from build123d import *

# Parameters (mm, degrees)
SKETCH1_R           = 2
BOSS_EXTRUDE1_DEPTH = 6
SKETCH2_R           = 10
BOSS_EXTRUDE2_DEPTH = 51
SKETCH3_R           = 7.75
CUT_EXTRUDE1_DEPTH  = 62.558024733
FILLET1_R           = 1


with BuildPart() as part:
    # Sketch1 → Boss-Extrude1 (new body)
    with BuildSketch(Plane(origin=(0, 0, 0), x_dir=(1, 0, 0), z_dir=(0, 1, 0))):
        Polygon((-16.274775851, 13.401142209), (-14.274775851, 15.401142209), (13.725224149, 15.401142209), (15.725224149, 13.401142209), (15.725224149, -14.598857791), (13.725224149, -16.598857791), (-14.274775851, -16.598857791), (-16.274775851, -14.598857791), align=None)
        with Locations(Location((11.038932647, 10.714850708, 0), (0, 0, 270))):
            Circle(SKETCH1_R, mode=Mode.SUBTRACT)
        with Locations(Location((-11.58848435, 10.714850708, 0), (0, 0, 270))):
            Circle(SKETCH1_R, mode=Mode.SUBTRACT)
        with Locations(Location((-11.58848435, -11.91256629, 0), (0, 0, 270))):
            Circle(SKETCH1_R, mode=Mode.SUBTRACT)
        with Locations(Location((11.038932647, -11.91256629, 0), (0, 0, 270))):
            Circle(SKETCH1_R, mode=Mode.SUBTRACT)
    extrude(amount=BOSS_EXTRUDE1_DEPTH)

    # Sketch2 → Boss-Extrude2 (add)
    with BuildSketch(Plane(origin=(0, 6, 0), x_dir=(1, 0, 0), z_dir=(0, 1, 0))):
        with Locations(Location((-0.274775851, -0.598857791, 0), (0, 0, 90))):
            Circle(SKETCH2_R)
    extrude(amount=BOSS_EXTRUDE2_DEPTH)

    # Sketch3 → Cut-Extrude1 (cut, through all)
    with BuildSketch(Plane(origin=(0, 57, 0), x_dir=(1, 0, 0), z_dir=(0, 1, 0))):
        with Locations(Location((-0.274775851, -0.598857791, 0), (0, 0, 270))):
            Circle(SKETCH3_R)
    extrude(amount=-CUT_EXTRUDE1_DEPTH, mode=Mode.SUBTRACT)

    # Fillet1
    fillet1_edges = [part.edges().sort_by_distance(p)[0] for p in [
        (-0.274775851, 6, 10.598857791),
    ]]
    fillet(fillet1_edges, radius=FILLET1_R)


solid = part.part
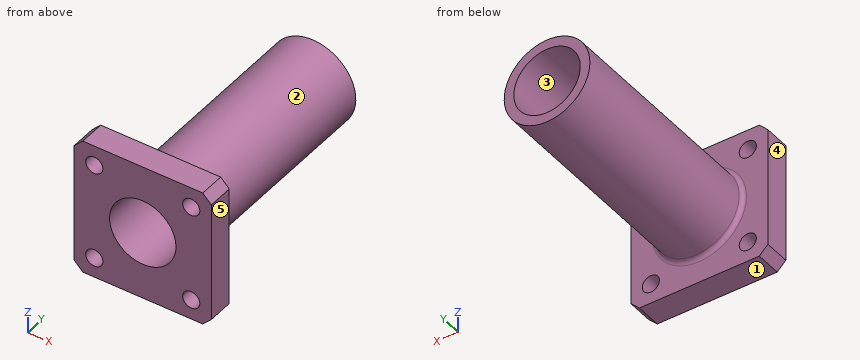
Could you check a few things on this model? Use its own coordinates, in mm. Face numbers are marked on the shaded views. A direction names the side the tool comes from. Coordinates: 2 decimals unless noted, no trailing zeros. Order: outer loops, then holes, each group sorted by start corner. A loop starts at its lowest first (then second) coordinate and runs counter-clockwise, first axis right, second up. Notation, with made-up numbers: (43.5, -34.5) - (57.5, -34.5) arc R21 cw to (57.5, -0.5) - close; hole circle Ø11 at (81, -15.5). An arc over 180 degrees is marked (long way). Answer in a Markdown table with one row per item. Add a question column.
(1) If we mould it in two halves opening along X, with no side actions, what happens to the marked faces 3, 4 and 5? For each: released by +X, released by -X, zero draft, split by the parting line, or undercut.
(2) If we section it at A-A, the plane x = -12.5: Please give me the cut outline in (y, z), then the cut area to 3 significant figures.
(3) Will these pins go through, and if not, where does the flat tip stop? pin 1 (2.5 mm diameter, centred on x = 11.04, z = 11.91, fed in from -Y); pin 2 (2 mm diameter, centred on y = 28.5, z = 7, fed in from -X); pin 3 (1.5 mm diameter, centred on y = 38.5, z = 3.5, fed in from -X); pin 4 (4 mm diameter, centred on y = 27, z = -10.5, fed in from -X).
(4) I need wall thicknesses on L1, parallel to Z at x = 0, y = 4; L2, parallel to X at y = 45, z = 1; L3, parallel to Y at x = 5, z = -11. Which ranges of each line are inside material? Lowest first, please.
(5) If we section it at B-B, the plane y = 21.5: Please give me the cut outline in (x, z), then the cut area to 3 significant figures.
(6) On a 3-axis mill with a long thin cutter (end or side, diameter ignored), from which of +Z, -Z, +X, -X, +Y, -Y can I reach the whole of each face in a straight line? I mean the marked faces 1 and 2. Say none if no direction works.
Results are:
| question | item | result |
|---|---|---|
| 1 | face 3 | undercut |
| 1 | face 4 | released by -X |
| 1 | face 5 | released by +X |
| 2 | outline | (0, -15.4) - (6, -15.4) - (6, -12.5) - (0, -12.5) - close; (0, -8.93) - (6, -8.93) - (6, 10.13) - (0, 10.13) - close; (0, 13.69) - (6, 13.69) - (6, 16.6) - (0, 16.6) - close |
| 2 | area | 149 mm2 |
| 3 | pin 1 | passes through |
| 3 | pin 2 | stops at x = -8.69 |
| 3 | pin 3 | stops at x = -10.04 |
| 3 | pin 4 | stops at x = -4.42 |
| 4 | L1 | z = -15.4 to -7.15, 8.34 to 16.6 |
| 4 | L2 | x = -10.27 to -8.01, 7.46 to 9.72 |
| 4 | L3 | y = 0 to 6 |
| 5 | outline | circle Ø20 at (-0.27, 0.6); hole circle Ø15.5 at (-0.27, 0.6) |
| 5 | area | 125 mm2 |
| 6 | face 1 | -Z, +X, -X, +Y, -Y |
| 6 | face 2 | +Y |
